from build123d import *

# Parameters (mm, degrees)
SKETCH1_R           = 15.5575
BOSS_EXTRUDE1_DEPTH = 1.524
SKETCH2_R           = 14.2875
BOSS_EXTRUDE2_DEPTH = 6.4008
SKETCH3_R           = 6.35
CUT_EXTRUDE1_DEPTH  = 24.38533873
FILLET1_R           = 0.254


with BuildPart() as part:
    # Sketch1 → Boss-Extrude1 (new body)
    with BuildSketch(Plane(origin=(0, 0, 0), x_dir=(0, 0, -1), z_dir=(1, 0, 0))):
        with Locations(Location((0, 0, 0), (0, 0, 180))):
            Circle(SKETCH1_R)
    extrude(amount=BOSS_EXTRUDE1_DEPTH)

    # Sketch2 → Boss-Extrude2 (add)
    with BuildSketch(Plane(origin=(1.524, 0, 0), x_dir=(0, 0, -1), z_dir=(1, 0, 0))):
        Circle(SKETCH2_R)
    extrude(amount=BOSS_EXTRUDE2_DEPTH)

    # Sketch3 → Cut-Extrude1 (cut, through all)
    with BuildSketch(Plane(origin=(7.9248, 0, 0), x_dir=(0, 0, -1), z_dir=(1, 0, 0))):
        Circle(SKETCH3_R)
    extrude(amount=-CUT_EXTRUDE1_DEPTH, mode=Mode.SUBTRACT)

    # Fillet1
    fillet1_edges = [part.edges().sort_by_distance(p)[0] for p in [
        (0, 0, -15.5575),
        (1.524, 0, -15.5575),
        (1.524, 0, 14.2875),
        (7.9248, 0, 14.2875),
    ]]
    fillet(fillet1_edges, radius=FILLET1_R)


solid = part.part
Part model, mm, in its own coordinate system. Give positions to 0.01 mm unless a question says otherwise; leave off trailing zeros. Loops run counter-clockwise (first coordinate to the right, second up) from the corner with the lowest first, then second, coordinate; pieces in that order, holes last. Notation, with made-up numbers: M -4,80 L 1,80 A33 cw 1,119 Z; hole C 17.25,57.25 d2. An arc over 180 degrees is marked long. Put each result on its own line as item: value. Start each with the question number.
1) Probe probe 1 along Y at (x, z) = (4.75, 0); probe 2 along Y at (x, z) = (5, 4.5); probe 3 along Z at (x, y) = (5, -5.5). List the from-to ranges inside material, lowest first.
2) Saw through at A-A (y = 0). List the corners of the cut face in (x, z), then the cut area to 3 significant figures.
3) Flat gauge pins, fed straight in: pin 1 (1.5 mm diameter, centred on x = 5, y = -3.5, fed in from +Z); pin 2 (1 mm diameter, centred on x = 2.5, y = 3, fed in from -Z); pin 3 (1.5 mm diameter, centred on y = -4.5, z = -3, fed in from -X); pin 4 (1 mm diameter, centred on x = 1, y = 3, fed in from +Z). Where does each tip first touch, or does it go through?
4) Pull direction Y, two halves, no side cores. Call faces 1 (the cylindrical face through (4.02, -6.2, 1.38)), 2 (the flat face through (1.524, 12.4, 7.9)), 3 (the cylindrical face through (4.683, 0.628, 14.274)): +Y half, -Y half, draft (parallel to the pull), parting line (faces both ways), or undercut.
Numbers:
1. probe 1: -14.29 to -6.35, 6.35 to 14.29
1. probe 2: -13.56 to -4.48, 4.48 to 13.56
1. probe 3: -13.19 to -3.17, 3.17 to 13.19
2. outline: M 0,-15.3 A0.25 ccw 0.25,-15.56 L 1.27,-15.56 A0.25 ccw 1.52,-15.3 L 1.52,-14.54 A0.25 cw 1.78,-14.29 L 7.67,-14.29 A0.25 ccw 7.92,-14.03 L 7.92,-6.35 L 0,-6.35 Z; M 0,6.35 L 7.92,6.35 L 7.92,14.03 A0.25 ccw 7.67,14.29 L 1.78,14.29 A0.25 cw 1.52,14.54 L 1.52,15.3 A0.25 ccw 1.27,15.56 L 0.25,15.56 A0.25 ccw 0,15.3 Z
2. area: 130 mm^2
3. pin 1: z = 14.02
3. pin 2: z = -14.07
3. pin 3: through
3. pin 4: z = 15.36
4. face 1: undercut
4. face 2: draft
4. face 3: parting line
